CAD build for the part. Positions are in the model's coordinates, mm. Face numbers are marked on the shaded views. A direction names the side the tool comes from. Coordinates: 2 decimals unless noted, no trailing zeros. Write each loop counter-clockwise with the first axis right and the second up, starting at its lowest first coordinate (ties: lowest second). Pieces come first, ordered by that corner, then holes. Notation, with made-up numbers: (-37.75, -36) -> (-0.75, -36) arc R21 ccw to (-0.75, -12) -> close; hole circle Ø11 at (4.5, -37). An arc over 180 degrees is marked (long way). Answer as CSV lines item,"result".
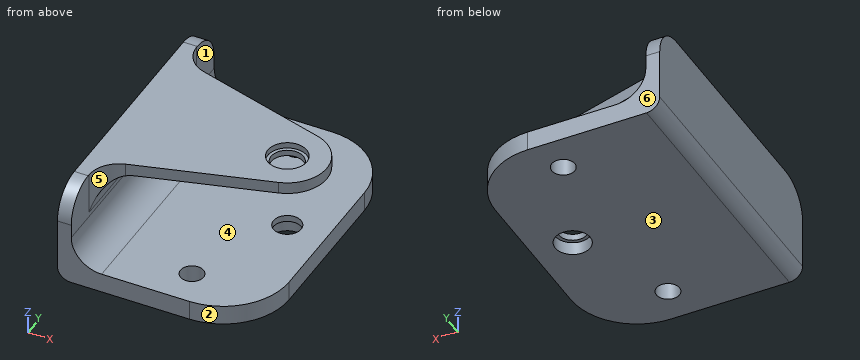
```python
from build123d import *

# Parameters (mm, degrees)
F1_DEPTH      = 26.8605
F2_R          = 2.667
F2_R_2        = 2.2225
F3_DEPTH      = 3.811
F3_DEPTH_BACK = 14.86
F4_R          = 2.2225
F5_DEPTH      = 2.286
F6_R          = 3.7465
F6_R_2        = 2.667
F7_DEPTH      = 1.143
F8_R          = 5.842
F9_R          = 6.35
F10_R         = 12.7
F11_R         = 2.54
F12_R         = 3.1115
F12_R_2       = 2.667
F13_DEPTH     = 1.143
F14_R         = 3.3655
F14_R_2       = 2.667
F15_DEPTH     = 2.54


with BuildPart() as f1:
    # F0 (on Front) → F1 (new body, symmetric)
    with BuildSketch(Plane.XZ):
        Polygon((0, 0), (38.1, 0), (38.1, 3.81), (2.667, 3.81), (2.667, 16.383), (38.1, 16.383), (38.1, 18.669), (0, 18.669), align=None)
    extrude(amount=F1_DEPTH, both=True)

    # F2 (on face) → F3 (cut, two sides)
    with BuildSketch(Plane.XY.offset(3.81)) as f3_sk:
        with Locations((30.48, 0)):
            Circle(F2_R)
        with Locations((22.225, 19.685)):
            Circle(F2_R_2)
        with Locations((22.225, -19.685)):
            Circle(F2_R_2)
    extrude(amount=-F3_DEPTH, mode=Mode.SUBTRACT)
    extrude(f3_sk.sketch, amount=F3_DEPTH_BACK, mode=Mode.SUBTRACT)

    # F4 (on face) → F5 (cut, through all)
    with BuildSketch(Plane.XY.offset(18.669)):
        with BuildLine():
            ThreePointArc((32.5741697301, 7.3265853671), (36.5636655621, 4.5883998658), (38.1, 0))
            Line((38.1, 0), (38.1, 26.8605))
            Line((38.1, 26.8605), (2.667, 26.8605))
            Line((2.667, 26.8605), (2.667, 15.875))
            Line((2.667, 15.875), (32.5741697301, 7.3265853671))
        make_face()
        with Locations((22.225, 19.685)):
            Circle(F4_R, mode=Mode.SUBTRACT)
        with BuildLine():
            Line((38.1, -26.8605), (38.1, 0))
            ThreePointArc((38.1, 0), (36.5636655621, -4.5883998658), (32.5741697301, -7.3265853671))
            Line((32.5741697301, -7.3265853671), (2.667, -15.875))
            Line((2.667, -15.875), (2.667, -26.8605))
            Line((2.667, -26.8605), (38.1, -26.8605))
        make_face()
        with Locations((22.225, -19.685)):
            Circle(F4_R, mode=Mode.SUBTRACT)
    extrude(amount=-F5_DEPTH, mode=Mode.SUBTRACT)

    # F6 (on face) → F7 (cut)
    with BuildSketch(Plane.XY.offset(18.669)):
        with Locations((30.48, 0)):
            Circle(F6_R)
        with Locations((30.48, 0)):
            Circle(F6_R_2, mode=Mode.SUBTRACT)
    extrude(amount=-F7_DEPTH, mode=Mode.SUBTRACT)

    # F8
    f8_edges = [f1.edges().sort_by_distance(p)[0] for p in [
        (2.667, 0, 3.81),
        (2.667, 0, 16.383),
        (2.667, 15.875, 17.526),
        (2.667, -15.875, 17.526),
    ]]
    fillet(f8_edges, radius=F8_R)

    # F9
    f9_edges = [f1.edges().sort_by_distance(p)[0] for p in [
        (1.3335, 26.8605, 18.669),
        (1.3335, -26.8605, 18.669),
    ]]
    fillet(f9_edges, radius=F9_R)

    # F10
    f10_edges = [f1.edges().sort_by_distance(p)[0] for p in [
        (38.1, 26.8605, 1.905),
        (38.1, -26.8605, 1.905),
    ]]
    fillet(f10_edges, radius=F10_R)

    # F11
    f11_edges = [f1.edges().sort_by_distance(p)[0] for p in [
        (0, 0, 0),
    ]]
    fillet(f11_edges, radius=F11_R)

    # F12 (on face) → F13 (cut, through all)
    with BuildSketch(Plane.XY.offset(17.526)):
        with Locations((30.48, 0)):
            Circle(F12_R)
        with Locations((30.48, 0)):
            Circle(F12_R_2, mode=Mode.SUBTRACT)
    extrude(amount=-F13_DEPTH, mode=Mode.SUBTRACT)

    # F14 (on face) → F15 (cut)
    with BuildSketch(Plane(origin=(0, 0, 0), x_dir=(1, 0, 0), z_dir=(0, 0, -1))):
        with Locations((30.48, 0)):
            Circle(F14_R)
        with Locations((30.48, 0)):
            Circle(F14_R_2, mode=Mode.SUBTRACT)
    extrude(amount=-F15_DEPTH, mode=Mode.SUBTRACT)


solid = f1.part
```
Item 1: Wall check: line 1 (Z direction, x = 17.5, y = 0); line 2 (X direction, y = 0, z = 3.1); line 3 (Z direction, x = 35.5, y = 19). Give the ranges that are in metal, low to high. Write a range as from..to.
Answer below:
line 1,"z = 0..3.81, 16.38..18.67"
line 2,"x = 0..27.81, 33.15..38.1"
line 3,"z = 0..3.81"
Item 2: Two-plate mould, pull along Z, no slides. Class the marked faces 1, 2 and 3: pulls with the +Z half, pulls with the -Z half, needs draft (parallel to the pull), parting line crosses it, or undercut.
Answer below:
face 1,"undercut"
face 2,"needs draft"
face 3,"pulls with the -Z half"
Item 3: Saw through at A-A on y = 0. Give the cut face in (x, z).
Answer below:
outline,"(0, 2.54) arc R2.54 ccw to (2.54, 0) -> (27.11, 0) -> (27.11, 2.54) -> (27.81, 2.54) -> (27.81, 3.81) -> (8.51, 3.81) arc R5.84 cw to (2.67, 9.65) -> (2.67, 10.54) arc R5.84 cw to (8.51, 16.38) -> (27.37, 16.38) -> (27.37, 17.53) -> (26.73, 17.53) -> (26.73, 18.67) -> (0, 18.67) -> close; (33.15, 2.54) -> (33.85, 2.54) -> (33.85, 0) -> (38.1, 0) -> (38.1, 3.81) -> (33.15, 3.81) -> close; (33.59, 16.38) -> (38.1, 16.38) -> (38.1, 18.67) -> (34.23, 18.67) -> (34.23, 17.53) -> (33.59, 17.53) -> close"
Item 4: Flat gauge pins, fed straight in: pin 1 (2 mm diameter, centred on y = -6, z = 6.5, fed in from +X); pin 2 (5 mm diameter, centred on x = 25.5, z = 16.5, fed in from +Y); pin 3 (6 mm diameter, centred on x = 30.48, y = 0, fed in from -Z). Where does each tip first touch, or does it go through?
Answer below:
pin 1,"stops at x = 4.4"
pin 2,"stops at y = 10.06"
pin 3,"stops at z = 2.54"
Item 5: Saw through at B-B on x = 16. Give the cut face in (y, z), and give its area (3 significant figures).
Answer below:
outline,"(-26.86, 0) -> (26.86, 0) -> (26.86, 3.81) -> (-26.86, 3.81) -> close; (-12.06, 16.38) -> (12.06, 16.38) -> (12.06, 18.67) -> (-12.06, 18.67) -> close"
area,"260 mm2"
Item 6: Saw through at D-D on z = 13.5. Give the cut face in (x, y), and give its area (3 significant figures).
Answer below:
outline,"(0, -26.75) -> (2.67, -26.75) -> (2.67, -20.28) arc R5.84 cw to (3.47, -17.32) -> (3.47, 17.32) arc R5.84 cw to (2.67, 20.28) -> (2.67, 26.75) -> (0, 26.75) -> close"
area,"172 mm2"
Item 7: 3-axis set-ups, long thin cutter, end or side, ignore diameter. For the marked faces 4, 5 and 6: which of +Z, -Z, +X, -X, +Y, -Y reach the whole face in a straight line?
Answer below:
face 4,"+X, +Y, -Y"
face 5,"+Z, +X, -Y"
face 6,"+Z, -Z, +X, -X, +Y"
Item 8: Saw through at C-C on x = 30.48. Give the cut face in (y, z), and give its area (3 significant figures).
Answer below:
outline,"(-25.8, 0) -> (-3.37, 0) -> (-3.37, 2.54) -> (-2.67, 2.54) -> (-2.67, 3.81) -> (-25.8, 3.81) -> close; (-7.93, 16.38) -> (-3.11, 16.38) -> (-3.11, 17.53) -> (-3.75, 17.53) -> (-3.75, 18.67) -> (-7.93, 18.67) -> close; (2.67, 2.54) -> (3.37, 2.54) -> (3.37, 0) -> (25.8, 0) -> (25.8, 3.81) -> (2.67, 3.81) -> close; (3.11, 16.38) -> (7.93, 16.38) -> (7.93, 18.67) -> (3.75, 18.67) -> (3.75, 17.53) -> (3.11, 17.53) -> close"
area,"193 mm2"
